The listing builds one solid part. Answer for the finished solid, in the listing's coordinates (mm). A direction names the side the tool comes from. Coordinates: 2 decimals unless noted, no trailing zeros. Order: outer loops, then holes, each group sorted by start corner. A loop starts at its lowest first (then second) coordinate and runs counter-clockwise, first axis right, second up. Notation, with made-up numbers: (40, 7.25) - (67, 7.25) arc R12 cw to (67, 21.25) - close; hole circle Ø8 at (-23.75, -1.75). An arc over 180 degrees is marked (long way). One line per item, written item: value. Start each with the question number.
Autodesk Inventor part; units mm, degrees
ref_plane "YZ Plane" through (0, 0, 0) normal (1, 0, 0) x (0, 1, 0)
ref_plane "XZ Plane" through (0, 0, 0) normal (0, 1, 0) x (-1, 0, 0)
ref_plane "XY Plane" through (0, 0, 0) normal (0, 0, 1) x (1, 0, 0)
sketch "Boceto1" plane through (0, 0, 0) normal (0, 0, 1) x (1, 0, 0)
  line L0 (0, 0) -> (0, 15)
  line L1 (0, 15) -> (2, 15)
  line L2 (2, 15) -> (8, 4.6077)
  line L3 (2, 15) -> (14, 15) construction
  line L4 (0, 0) -> (0, -5)
  line L5 (8, 4.6077) -> (14, 4.6077)
  line L6 (14, 4.6077) -> (20, 15)
  line L7 (20, 15) -> (22, 15)
  line L8 (22, 15) -> (22, -0.0111)
  line L9 (22, -0.0111) -> (22, -5)
  line L10 (22, -5) -> (0, -5)
  dimension "d0" = 15
  dimension "d1" = 2
  dimension "d2" = 12
  dimension "d3" = 60
  dimension "d4" = 5
  dimension "d5" = 6
  dimension "d6" = 12
  dimension "d7" = 2
extrude "Extrusión1" add sketch "Boceto1" along normal blind 15
sketch "Boceto2" plane through (0, 0, 15) normal (0, 0, 1) x (1, 0, 0)
  line L0 (14, 4.6077) -> (8, 4.6077)
  line L1 (8, 4.6077) -> (9, 4.6077)
  line L2 (9, 4.6077) -> (9, -1.3923)
  line L3 (9, -1.3923) -> (13, -1.3923)
  line L4 (13, -1.3923) -> (13, 4.6077)
  line L5 (9, 4.6077) -> (13, 4.6077)
  point P0 (0, 0)
  dimension "d10" = 1
  dimension "d11" = 6
  dimension "d12" = 4
extrude "Extrusión2" cut sketch "Boceto2" against normal blind 12
sketch "Boceto3" plane through (0, 0, 0) normal (0, 0, -1) x (-1, 0, 0)
  line L0 (-22, -5) -> (-22, 15)
  line L1 (-22, -5) -> (-22, 15)
  line L2 (-2, 15) -> (0, 15)
  line L3 (-22, 15) -> (0, 15)
  line L4 (0, 15) -> (0, -5)
  line L5 (0, 15) -> (0, -5)
  line L6 (0, -5) -> (-22, -5)
  line L7 (0, -5) -> (-22, -5)
  line L8 (-16.5, 0) -> (-15, 0)
  line L9 (-16.5, 0) -> (-18, 0)
  line L10 (-11, 11) -> (-12.5, 11)
  line L11 (-12.5, 11) -> (-18, 0)
  line L12 (-11, 11) -> (-9.5, 11)
  line L13 (-5.5, 0) -> (-7, 0)
  line L14 (-5.5, 0) -> (-4, 0)
  line L15 (-4, 0) -> (-9.5, 11)
  line L16 (-15, 0) -> (-14, 2)
  line L17 (-7, 0) -> (-8, 2)
  line L18 (-14, 2) -> (-8, 2)
  line L19 (-11, 4) -> (-10, 4)
  line L20 (-10, 4) -> (-9, 4)
  line L21 (-9, 4) -> (-11, 8)
  line L22 (-11, 4) -> (-13, 4)
  line L23 (-13, 4) -> (-11, 8)
  line L24 (-13, 4) -> (-11, 8)
  line L25 (-11, 8) -> (-9, 4)
  line L26 (-9, 4) -> (-13, 4)
  point P0 (0, 0)
  dimension "d16" = 1.5
  dimension "d23" = 1.5
  dimension "d24" = 1.5
  dimension "d25" = 1.5
  dimension "d26" = 3
  dimension "d27" = 4
  dimension "d29" = 1
extrude "Extrusión3" add sketch "Boceto3" against normal blind 3 contours L0 L3 L2 L4 L6 | L9 L11 L10 L12 L15 L14 L13 L17 L18 L16 L8 | L22 L23 L21 L20 L19
extrude "Extrusión4" cut sketch "Boceto3" against normal blind 1 contours L9 L11 L10 L12 L15 L14 L13 L17 L18 L16 L8
properties part number "soporte_antena_aquiles"
(1) The part is cut by section B-B on y = 3.5. Determine the outline of the cut face in (x, z), plus the area to 4 significant figures.
(2) For a pull along X with two mould halves and no side action, classify faces 1 (the face through (11, 1, 0)), 2 (the face through (22, 5, 7)), 3 (the face through (11, 9, 3)) as pulls with the +X half, pulls with the -X half, needs draft (parallel to the pull), parting line crosses it, or undercut.
(3) Consider probe 1 along X at (y, z) = (2.25, 3.75); probe 2 along Z at (x, y) = (5.25, 9.5); probe 3 along Z at (x, y) = (13.25, 9). Determine where each line is inside the solid, lowest interval first.
(4) Flat-ended cylindrical pins translate along their axes: pin 1 Ø1.2 at (x, z) = (12, 11.5) entering from +Y; pin 2 Ø0.8 at (x, z) = (13.5, 10.5) entering from +Y; pin 3 Ø5 at (x, z) = (17, 12.5) entering from +Y. Find the tip coordinate at first contact, or state that the pin passes through.
(5) The part is cut by section A-A on x = 11.5. Determine the outline of the cut face in (y, z).
(6) The part is cut by section D-D on x = 6. Determine the outline of the cut face in (y, z).
(7) For faces 4 (the face through (0, 5, 7)), 5 (the face through (8.5, 4.608, 8.9)), 6 (the face through (6.7, 5.4, 0.5)), determine the directions among +Z, -Z, +X, -X, +Y, -Y from which every point of the face is accessible in a straight line to the end or side of a thin tool.
(8) The part is cut by section C-C on z = 5. Determine the outline of the cut face in (x, y), plus the area to 3 significant figures.
Completed:
1. outline: (0, 0) - (5.75, 0) - (5.75, 1) - (16.25, 1) - (16.25, 0) - (22, 0) - (22, 15) - (13, 15) - (13, 3) - (9, 3) - (9, 15) - (0, 15) - close
1. area: 271.5 mm2
2. face 1: needs draft
2. face 2: pulls with the +X half
2. face 3: undercut
3. probe 1: x = 0 to 9, 13 to 22
3. probe 2: z = 0 to 3
3. probe 3: z = 1 to 3
4. pin 1: stops at y = -1.39
4. pin 2: stops at y = 4.61
4. pin 3: stops at y = 14.13
5. outline: (-5, 0) - (2, 0) - (2, 1) - (4, 1) - (4, 0) - (7, 0) - (7, 1) - (11, 1) - (11, 0) - (15, 0) - (15, 3) - (-1.39, 3) - (-1.39, 15) - (-5, 15) - close
6. outline: (-5, 0) - (0, 0) - (0, 1) - (4, 1) - (4, 0) - (15, 0) - (15, 3) - (8.07, 3) - (8.07, 15) - (-5, 15) - close
7. face 4: +Z, -Z, -X, +Y, -Y
7. face 5: +Z, +Y
7. face 6: -Z
8. outline: (0, -5) - (22, -5) - (22, 15) - (20, 15) - (14, 4.61) - (13, 4.61) - (13, -1.39) - (9, -1.39) - (9, 4.61) - (8, 4.61) - (2, 15) - (0, 15) - close
8. area: 291 mm2
